Check sheet for the drawn part. Datum: minimum x, y, z corner. Units: mm. Round coordinates to 2 decimals unless told otherwise and drop trailing zeros. Loops run counter-clockwise (first coordinate to the right, second up) from the corner with the lowest first, then second, coordinate; pieces in that order, holes last. Notation, with made-up numbers: (52.25, 89) -> (72.25, 89) arc R23 ccw to (72.25, 126) -> close; hole circle Ø10 at (2, 2.5). An arc over 180 degrees is marked (long way). Return JSON: item names as keys, results as strings.
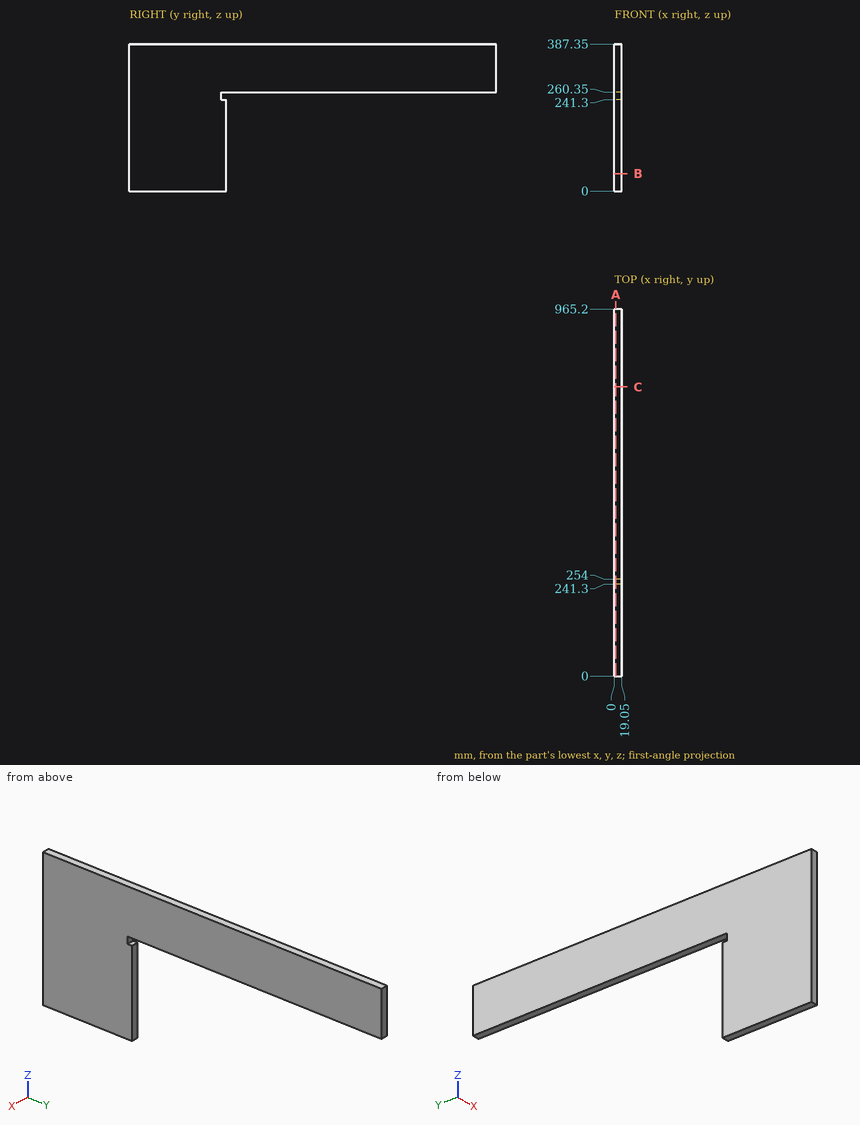
Q1. Section check C-C (y = 760.5). Record the boundary of the cut face in (x, z), then the cut area to 3 significant figures.
Results list:
{"outline": "(0, 260.35) -> (19.05, 260.35) -> (19.05, 387.35) -> (0, 387.35) -> close", "area": "2,420 mm^2"}
Q2. Section check A-A (x = 4.25). Record the boundary of the cut face in (y, z).
Results list:
{"outline": "(0, 0) -> (254, 0) -> (254, 241.3) -> (241.3, 241.3) -> (241.3, 260.35) -> (965.2, 260.35) -> (965.2, 387.35) -> (0, 387.35) -> close"}
Q3. Go/stop test with flat-tipped pins: pin 1 (8 mm diameter, centred on y = 108, z = 109.5, fed in from -X); pin 2 (5.5 mm diameter, centred on x = 13, z = 251, fed in from +Y); pin 3 (5.5 mm diameter, centred on x = 8, y = 605, fed in from -Z). Record where each tip stops, or that it passes through.
Results list:
{"pin 1": "x = 0", "pin 2": "y = 241.3", "pin 3": "z = 260.35"}
Q4. Material ranges on line 1 (Z direction, x = 4.25, y = 331.5); line 2 (Y direction, x = 1, z = 185); line 3 (Y direction, x = 10.25, z = 248.5), recorded low to high.
Results list:
{"line 1": "260.35 to 387.35", "line 2": "0 to 254", "line 3": "0 to 241.3"}
Q5. Section check B-B (z = 46.5). Record the boundary of the cut face in (x, y), then the cut area to 3 significant figures.
Results list:
{"outline": "(0, 0) -> (19.05, 0) -> (19.05, 254) -> (0, 254) -> close", "area": "4,840 mm^2"}
